```python
from build123d import *

# Parameters (mm, degrees)
SKETCH1_R               = 26
SKETCH1_R_2             = 2
SKETCH1_R_3             = 7.5
BOSS_EXTRUDE1_DEPTH     = 4
SKETCH3_R               = 9.75
SKETCH3_R_2             = 7.5
BOSS_EXTRUDE2_DEPTH     = 58
CUT_EXTRUDE1_DEPTH      = 73.083285164
CUT_EXTRUDE1_DEPTH_BACK = 73.083285164
SKETCH5_R               = 2.5
CUT_EXTRUDE2_DEPTH      = 73.08328525
CUT_EXTRUDE2_DEPTH_BACK = 73.08328525
SKETCH6_R               = 2.5


with BuildPart() as part:
    # Sketch1 → Boss-Extrude1 (new body)
    with BuildSketch(Plane(origin=(0, 0, 0), x_dir=(1, 0, 0), z_dir=(0, 1, 0))):
        with Locations(Location((0, 0, 0), (0, 0, 270))):
            Circle(SKETCH1_R)
        with Locations(Location((-12.5, 12.5, 0), (0, 0, 270))):
            Circle(SKETCH1_R_2, mode=Mode.SUBTRACT)
        with Locations(Location((-12.5, -12.5, 0), (0, 0, 270))):
            Circle(SKETCH1_R_2, mode=Mode.SUBTRACT)
        with Locations(Location((12.5, 12.5, 0), (0, 0, 270))):
            Circle(SKETCH1_R_2, mode=Mode.SUBTRACT)
        with Locations(Location((12.5, -12.5, 0), (0, 0, 270))):
            Circle(SKETCH1_R_2, mode=Mode.SUBTRACT)
        with Locations(Location((0, 0, 0), (0, 0, 270))):
            Circle(SKETCH1_R_3, mode=Mode.SUBTRACT)
    extrude(amount=BOSS_EXTRUDE1_DEPTH)

    # Sketch3 → Boss-Extrude2 (add)
    with BuildSketch(Plane(origin=(0, 4, 0), x_dir=(1, 0, 0), z_dir=(0, 1, 0))):
        with Locations(Location((0, 0, 0), (0, 0, 90))):
            Circle(SKETCH3_R)
        with Locations(Location((0, 0, 0), (0, 0, 270))):
            Circle(SKETCH3_R_2, mode=Mode.SUBTRACT)
    extrude(amount=BOSS_EXTRUDE2_DEPTH)

    # Sketch5 → Cut-Extrude1 (cut, two sides: drawn at the far end of the back side and taken through both)
    with BuildSketch(Plane.XY.offset(-CUT_EXTRUDE1_DEPTH_BACK)):
        with Locations((0, 35)):
            Circle(SKETCH5_R)
    extrude(amount=CUT_EXTRUDE1_DEPTH + CUT_EXTRUDE1_DEPTH_BACK, mode=Mode.SUBTRACT)

    # Sketch6 → Cut-Extrude2 (cut, two sides: drawn at the far end of the back side and taken through both)
    with BuildSketch(Plane(origin=(0, 0, 0), x_dir=(0, 0, -1), z_dir=(1, 0, 0)).offset(-CUT_EXTRUDE2_DEPTH_BACK)):
        with Locations((0, 51)):
            Circle(SKETCH6_R)
    extrude(amount=CUT_EXTRUDE2_DEPTH + CUT_EXTRUDE2_DEPTH_BACK, mode=Mode.SUBTRACT)


solid = part.part
```
Can you work these out from the model? Positions are in its coordinate system, mm. A direction names the side the tool comes from. Give positions to 0.01 mm unless a question says otherwise; leave off trailing zeros. Loops run counter-clockwise (first coordinate to the right, second up) from the corner with the lowest first, then second, coordinate; pieces in that order, holes last. Notation, with made-up numbers: M 7,52 L 18,52 A18 ccw 18,58 Z; hole C 3,37.5 d5. An arc over 180 degrees is marked long. Use CSV: the item, a comma, the result in double quotes. Start each with the question number.
1. Imagine slicing it at D-D, the plane z = 11.5. Write out the boundary of the cut face in (x, y).
2. On a 3-axis mill with a long thin cutter (end or side, diameter ignored), from which of +Z, -Z, +X, -X, +Y, -Y can I reach the whole of each face in a straight line? I mean faces 1 (the face through (-2.93, 32.59, -9.3)), 2 (the face through (6, 62, -5)). Say none if no direction works.
3. For P1, Ø6, axis at x = -17.5, z = -1, coming from the +Y side; P2, Ø8, axis at y = 8.5, z = 2, coming from the +X side; P3, Ø6.5, axis at y = 51, z = 0, coming from the -X side, each with a flat end and sliding along its axis, tell me the tip position at first contact or that it passes through.
4. If I drill on L1, parallel to X at y = 45, z = 0; L2, parallel to X at y = 2, z = -12, over which ranges is the centre line in solid material (lowest first)?
5. Imagine slicing it at B-B, the plane x = 0. Write out the boundary of the cut face in (y, z).
6. If we mould it in two halves opening along Y, with no side actions, what happens to faces 3 (the face through (-15.821, 1.972, -20.633)), 4 (the face through (-8.43, 48.78, -1.15)), 5 (the face through (0, 4, 11)), 6 (the face through (8.4, 50.04, -2.31))? For each: released by +Y, released by -Y, zero draft, split by the parting line, or undercut.
7. Imagine slicing it at C-C, the plane y = 51. Write out the boundary of the cut face in (x, z), plus the area to 3 significant figures.
8. Imagine slicing it at A-A, the plane z = 0. Write out the boundary of the cut face in (x, y), plus the area to 4 significant figures.
Response values:
1,outline,"M -23.32,0 L -14.23,0 L -14.23,4 L -23.32,4 Z; M -10.77,0 L 10.77,0 L 10.77,4 L -10.77,4 Z; M 14.23,0 L 23.32,0 L 23.32,4 L 14.23,4 Z"
2,face 1,"+Y"
2,face 2,"+Z, -Z, +X, -X, +Y"
3,P1,"y = 4"
3,P2,"x = 9.75"
3,P3,"x = -9.75"
4,L1,"-9.75 to -7.5, 7.5 to 9.75"
4,L2,"-23.07 to -14.44, -10.56 to 10.56, 14.44 to 23.07"
5,outline,"M 0,-26 L 4,-26 L 4,-9.75 L 32.5,-9.75 L 32.5,-7.5 L 0,-7.5 Z; M 0,7.5 L 32.5,7.5 L 32.5,9.75 L 4,9.75 L 4,26 L 0,26 Z; M 37.5,-9.75 L 62,-9.75 L 62,-7.5 L 37.5,-7.5 Z; M 37.5,7.5 L 62,7.5 L 62,9.75 L 37.5,9.75 Z"
6,face 3,"zero draft"
6,face 4,"undercut"
6,face 5,"released by +Y"
6,face 6,"undercut"
7,outline,"M -9.42,-2.5 A9.75 ccw 9.42,-2.5 L 7.07,-2.5 A7.5 cw -7.07,-2.5 Z; M -9.42,2.5 L -7.07,2.5 A7.5 cw 7.07,2.5 L 9.42,2.5 A9.75 ccw Z"
7,area,"99.1 mm^2"
8,outline,"M -26,0 L -7.5,0 L -7.5,48.5 L -9.75,48.5 L -9.75,4 L -26,4 Z; M -9.75,53.5 L -7.5,53.5 L -7.5,62 L -9.75,62 Z; M 7.5,0 L 26,0 L 26,4 L 9.75,4 L 9.75,48.5 L 7.5,48.5 Z; M 7.5,53.5 L 9.75,53.5 L 9.75,62 L 7.5,62 Z"
8,area,"386.5 mm^2"
